Input: part model. Units: mm. Frame: model coordinates. Face numbers are marked on the shaded views. A direction names the side the tool comes from. Give positions to 0.01 mm unless a question says otherwise; leave off trailing zeros. Order: outer loops, then holes, each group sorted by start corner. A loop starts at its lowest first (then second) coordinate and runs counter-clockwise, first axis right, second up.
```python
from build123d import *

# Parameters (mm, degrees)
BOSS_EXTRUDE1_DEPTH     = 2
BOSS_EXTRUDE2_DEPTH     = 96
BOSS_EXTRUDE3_DEPTH     = 2
CUT_EXTRUDE1_DEPTH      = 2
CUT_EXTRUDE2_DEPTH      = 20
CUT_EXTRUDE2_DEPTH_BACK = 2
SKETCH6_W               = 5
SKETCH6_H               = 10
CUT_EXTRUDE3_DEPTH      = 2


with BuildPart() as part:
    # Sketch1 → Boss-Extrude1 (new body)
    with BuildSketch(Plane(origin=(0, 0, 0), x_dir=(0, 0, -1), z_dir=(1, 0, 0))):
        Polygon((-46.565590075, -45.805369128), (3.434409925, -45.805369128), (-26.565590075, 54.194630872), (-46.565590075, 54.194630872), align=None)
    extrude(amount=BOSS_EXTRUDE1_DEPTH)

    # Sketch2 → Boss-Extrude2 (add)
    with BuildSketch(Plane(origin=(2, 0, 0), x_dir=(0, 0, -1), z_dir=(1, 0, 0))):
        Polygon((-26.565590075, 54.194630872), (3.434409925, -45.805369128), (-44.565590075, -45.805369128), (-46.565590075, -45.805369128), (-46.565590075, -43.805369128), (-44.565590075, -43.805369128), (0.746348624, -43.805369128), (-28.053651376, 52.194630872), (-44.565590075, 52.194630872), (-44.565590075, 54.194630872), align=None)
    extrude(amount=BOSS_EXTRUDE2_DEPTH)

    # Sketch3 → Boss-Extrude3 (add)
    with BuildSketch(Plane(origin=(98, 0, 0), x_dir=(0, 0, -1), z_dir=(1, 0, 0))):
        Polygon((-46.565590075, 54.194630872), (-26.565590075, 54.194630872), (3.434409925, -45.805369128), (-46.565590075, -45.805369128), align=None)
    extrude(amount=BOSS_EXTRUDE3_DEPTH)

    # Sketch4 → Cut-Extrude1 (cut)
    with BuildSketch(Plane(origin=(0, 54.194630872, 0), x_dir=(1, 0, 0), z_dir=(0, 1, 0))):
        Polygon((50, -30.815590075), (59, -30.815590075), (59, -36.565590075), (59, -42.315590075), (41, -42.315590075), (41, -30.815590075), align=None)
        Polygon((72.5, -30.815590075), (72.5, -42.315590075), (90.5, -42.315590075), (90.5, -36.565590075), (90.5, -30.815590075), align=None)
        Polygon((27.5, -30.815590075), (27.5, -42.315590075), (9.5, -42.315590075), (9.5, -36.565590075), (9.5, -30.815590075), align=None)
    extrude(amount=-CUT_EXTRUDE1_DEPTH, mode=Mode.SUBTRACT)

    # Sketch5 → Cut-Extrude2 (cut, two sides: drawn at the far end of the back side and taken through both)
    with BuildSketch(Plane.XY.offset(-CUT_EXTRUDE2_DEPTH_BACK)):
        Polygon((85, -11.305369128), (50, -11.305369128), (15, -11.305369128), (15, -20.805369128), (15, -30.305369128), (85, -30.305369128), align=None)
    extrude(amount=CUT_EXTRUDE2_DEPTH + CUT_EXTRUDE2_DEPTH_BACK, mode=Mode.SUBTRACT)

    # Sketch6 → Cut-Extrude3 (cut)
    with BuildSketch(Plane(origin=(100, 0, 0), x_dir=(0, 0, -1), z_dir=(1, 0, 0))):
        with Locations((-37.982930648, -35.987256773)):
            Rectangle(SKETCH6_W, SKETCH6_H)
    extrude(amount=-CUT_EXTRUDE3_DEPTH, mode=Mode.SUBTRACT)


solid = part.part
```
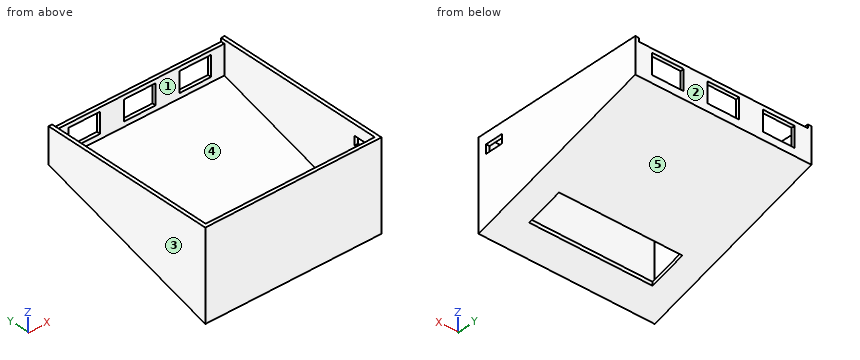
1) Cut plane C-C (x = 25). Return the cut outline in (y, z), then the cut area to 3 significant figures.
2) Reachability of the marked faces 1 and 2 from +Z, -Z, +X, -X, +Y, -Y: full face, straight path, thin tool, end or side. Return the list, or none.
3) Line query: probe 1 along X at (y, z) = (-38.5, 21); probe 2 along Y at (x, z) = (15, 43); probe 3 along Y at (x, z) = (82.5, 38). Output: solid intervals per line, ascending.
4) Cut plane D-D (z = 24.5). Return the cut outline in (x, y), then the cut area to 3 significant figures.
5) Cut plane A-A (x = 39.5). Return the cut outline in (y, z).
6) Cut plane B-B (y = -22). Return the cut outline in (x, z).
7) First-contact query: P1, Ø2, axis at x = 82.5, y = 53, coming from the +Z side; P2, Ø6, axis at x = 12.5, y = -31.5, coming from the -Z side; P3, Ø5, axis at x = 42, y = -11.5, coming from the +Z side. Flat tips, straight axial feed; report the tip coordinate or a pass-through.
8) Pull-direction query (Y, two-part tool) for the marked faces 3, 4 and 5; classes: pulls with the +Y half, pulls with the -Y half, needs draft (parallel to the pull), parting line crosses it, or undercut.
Geometry says:
1. outline: (-45.81, -3.43) - (-30.31, 1.22) - (-30.31, 3.3) - (-43.81, -0.75) - (-43.81, 46.57) - (-45.81, 46.57) - close; (-11.31, 6.92) - (54.19, 26.57) - (54.19, 30.82) - (52.19, 30.82) - (52.19, 28.05) - (-11.31, 9) - close; (52.19, 42.32) - (54.19, 42.32) - (54.19, 44.57) - (52.19, 44.57) - close
1. area: 274 mm2
2. face 1: +Z
2. face 2: +Z, -Z, +X, -X, +Y
3. probe 1: x = 0 to 2, 98 to 100
3. probe 2: y = -45.81 to -43.81, 52.19 to 54.19
3. probe 3: y = -45.81 to -43.81
4. outline: (0, -45.81) - (100, -45.81) - (100, 47.31) - (0, 47.31) - close; hole (2, -43.81) - (98, -43.81) - (98, 40.35) - (2, 40.35) - close
4. area: 1,230 mm2
5. outline: (-45.81, -3.43) - (-30.31, 1.22) - (-30.31, 3.3) - (-43.81, -0.75) - (-43.81, 46.57) - (-45.81, 46.57) - close; (-11.31, 6.92) - (54.19, 26.57) - (54.19, 44.57) - (52.19, 44.57) - (52.19, 28.05) - (-11.31, 9) - close
6. outline: (0, 3.71) - (15, 3.71) - (15, 5.8) - (2, 5.8) - (2, 46.57) - (0, 46.57) - close; (85, 3.71) - (100, 3.71) - (100, 46.57) - (98, 46.57) - (98, 5.8) - (85, 5.8) - close
7. P1: stops at z = 44.57
7. P2: stops at z = -0.04
7. P3: stops at z = 9.7
8. face 3: needs draft
8. face 4: undercut
8. face 5: pulls with the +Y half
